Can you work these out from the model? Positions are in its coordinate system, mm. A direction names the side the tool comes from. Coordinates: 2 decimals unless noted, no trailing zeros. Write each loop counter-clockwise with the first axis right and the second up, starting at its lowest first coordinate (ties: lowest second). Pieces come first, ordered by that corner, then holes. Notation, with made-up numbers: M 51,50 L 82,50 A21 cw 82,84 Z; hole C 52,-30.5 d2. An arc over 180 degrees is marked long. Answer as a JSON object with one key per item and string values. Group by question number.
Solid Edge part; units mm, degrees
sketch "Sketch1" plane through (0, 0, 0) normal (0, -1, 0) x (1, 0, 0)
  circle A0 centre (0, 0) radius 15
  circle A1 centre (0, 0) radius 9
extrude "Protrusion1" add sketch "Sketch1" against normal blind 10
sketch "Sketch2" plane through (0, 0, 0) normal (0, -1, 0) x (1, 0, 0)
  line L0 (-2, 8.775) -> (-2, 10)
  line L1 (-2, 10) -> (2, 10)
  line L2 (2, 10) -> (2, 8.775)
  arc A0 (2, 8.775) -> (8.8741, 1.5) centre (0, 0) cw
  line L3 (8.8741, 1.5) -> (10, 1.5)
  line L4 (10, 1.5) -> (10, -1.5)
  line L5 (10, -1.5) -> (8.8741, -1.5)
  line L6 (1.5, -10) -> (1.5, -8.8741)
  line L7 (-1.5, -10) -> (1.5, -10)
  line L8 (-1.5, -8.8741) -> (-1.5, -10)
  arc A1 (-1.5, -8.8741) -> (-8.8741, -1.5) centre (0, 0) cw
  line L9 (-10, -1.5) -> (-8.8741, -1.5)
  line L10 (-10, 1.5) -> (-10, -1.5)
  line L11 (-8.8741, 1.5) -> (-10, 1.5)
  arc A2 (-8.8741, 1.5) -> (-2, 8.775) centre (0, 0) cw
  line L12 (8.8741, -1.5) -> (1.5, -8.8741)
  dimension "D1" = 2
  dimension "D2" = 10
  dimension "D3" = 1.5
  dimension "D4" = 10
extrude "Extrusionsausschnitt_1" cut sketch "Sketch2" against normal blind 517
Q1. If we section it at D-D on x = -10.75: List the corners of the cut face in (y, z) for me.
Q2. If we section it at C-C on y = 6: List the corners of the cut face in (x, z) for me.
Q3. If we section it at B-B on x = 0: List the corners of the cut face in (y, z) for me.
Q4. If we section it at A-A on z = 0: List the corners of the cut face in (x, y) for me, and give its area (3 significant figures).
Q5. On a 3-axis mill with a long thin cutter (end or side, diameter ignored), from which of +Z, -Z, +X, -X, +Y, -Y can I reach the whole of each face in a straight line? I mean faces 1 (the flat face through (-10, 5, 0)), 2 (the flat face through (-6.5, 10, -6.5)). Say none if no direction works.
Q6. Will these pins go through, and if not, where does the flat tip stop? pin 1 (0.9 mm diameter, centred on x = -9.5, y = 5, fed in from +Z); pin 2 (2 mm diameter, centred on y = 7, z = -3.5, fed in from +X); pin 3 (0.9 mm diameter, centred on x = -9.5, y = 3, fed in from -Z).
Q7. Please list where these lines run through material, in increasing order: L1, parallel to Z at x = -0.25, y = 4; L2, parallel to Z at x = 5, y = 8.5; L3, parallel to X at y = 3.25, z = 3.
Q8. We'd pull the mould along Z, two halves only. Please class faces 3 (the cylindrical face through (-6.42, 4.93, -6.31)), 4 (the cylindrical face through (-14.985, 4.93, 0.66)), 5 (the flat face through (-6.5, 0, -6.5)), 6 (the cylindrical face through (6.59, 4.93, 6.13)): pulls with the +Z half, pulls with the -Z half, needs draft (parallel to the pull), parting line crosses it, or undercut.
Reply:
{
 "1": {"outline": "M 0,-10.46 L 10,-10.46 L 10,10.46 L 0,10.46 Z"},
 "2": {"outline": "C 0,0 d30; hole M -10,-1.5 L -8.87,-1.5 A9 ccw -1.5,-8.87 L -1.5,-10 L 1.5,-10 L 1.5,-8.87 A9 ccw 8.87,-1.5 L 10,-1.5 L 10,1.5 L 8.87,1.5 A9 ccw 2,8.77 L 2,10 L -2,10 L -2,8.77 A9 ccw -8.87,1.5 L -10,1.5 Z"},
 "3": {"outline": "M 0,-15 L 10,-15 L 10,-10 L 0,-10 Z; M 0,10 L 10,10 L 10,15 L 0,15 Z"},
 "4": {"outline": "M -15,0 L -10,0 L -10,10 L -15,10 Z; M 10,0 L 15,0 L 15,10 L 10,10 Z", "area": "100 mm^2"},
 "5": {"face 1": "+Y, -Y", "face 2": "+Z, -Z, +X, -X, +Y"},
 "6": {"pin 1": "z = 11.96", "pin 2": "x = 14.79", "pin 3": "z = -11.96"},
 "7": {"L1": "-15 to -10, 10 to 15", "L2": "-14.14 to -7.48, 7.48 to 14.14", "L3": "-14.7 to -8.49, 8.49 to 14.7"},
 "8": {"face 3": "undercut", "face 4": "parting line crosses it", "face 5": "needs draft", "face 6": "undercut"}
}
